from build123d import *

# Parameters (mm, degrees)
F0_W     = 76.2
F0_H     = 76.2
F1_DEPTH = 76.2
F2_T     = -7.62
F3_W     = 60.96
F3_H     = 60.96
F4_DEPTH = 25.4
F5_W     = 60.96
F5_H     = 60.96
F6_DEPTH = 25.4
F7_W     = 60.96
F7_H     = 60.96
F8_DEPTH = 25.4


with BuildPart() as f1:
    # F0 (on Top) → F1 (new body)
    with BuildSketch(Plane.XY):
        with Locations((-3.61854, -0.157197)):
            Rectangle(F0_W, F0_H)
    extrude(amount=F1_DEPTH)

    # F2
    f2_openings = [f1.faces().sort_by_distance(p)[0] for p in [
        (-3.61854, -38.257197, 38.1),
    ]]
    offset(amount=F2_T, openings=f2_openings)

    # F3 (on face) → F4 (cut)
    with BuildSketch(Plane(origin=(-41.71854, 0, 0), x_dir=(0, -1, 0), z_dir=(-1, 0, 0))):
        with Locations((0.157197, 38.1)):
            Rectangle(F3_W, F3_H)
    extrude(amount=-F4_DEPTH, mode=Mode.SUBTRACT)

    # F5 (on face) → F6 (cut)
    with BuildSketch(Plane(origin=(0, 37.942803, 0), x_dir=(-1, 0, 0), z_dir=(0, 1, 0))):
        with Locations((3.61854, 38.1)):
            Rectangle(F5_W, F5_H)
    extrude(amount=-F6_DEPTH, mode=Mode.SUBTRACT)

    # F7 (on face) → F8 (cut)
    with BuildSketch(Plane.YZ.offset(34.48146)):
        with Locations((-0.157197, 38.1)):
            Rectangle(F7_W, F7_H)
    extrude(amount=-F8_DEPTH, mode=Mode.SUBTRACT)


solid = f1.part
CAD build for the part. Positions are in the model's coordinates, mm. A direction names the side the tool comes from. Coordinates: 2 decimals unless noted, no trailing zeros. Order: outer loops, then holes, each group sorted by start corner. A loop starts at its lowest first (then second) coordinate and runs counter-clockwise, first axis right, second up.
Item 1: Band-saw the part on C-C on z = 9.5. List the corners of the cut face in (x, y), plus the area to 3 significant figures.
Check sheet entries:
outline: (-41.72, -38.26) - (-34.1, -38.26) - (-34.1, -30.64) - (-41.72, -30.64) - close; (-41.72, 30.32) - (-34.1, 30.32) - (-34.1, 37.94) - (-41.72, 37.94) - close; (26.86, -38.26) - (34.48, -38.26) - (34.48, -30.64) - (26.86, -30.64) - close; (26.86, 30.32) - (34.48, 30.32) - (34.48, 37.94) - (26.86, 37.94) - close
area: 232 mm2
Item 2: Drill centre lines: L1, parallel to Z at x = -21, y = -16; L2, parallel to X at y = -31.5, z = 30.5; L3, parallel to Y at x = 28, z = 55.5. Where is each one in solid material? Low to high.
Check sheet entries:
L1: z = 0 to 7.62, 68.58 to 76.2
L2: x = -41.72 to -34.1, 26.86 to 34.48
L3: y = -38.26 to -30.64, 30.32 to 37.94
Item 3: Band-saw the part on A-A on y = 11.5. List the corners of the cut face in (x, z).
Check sheet entries:
outline: (-41.72, 0) - (34.48, 0) - (34.48, 7.62) - (-41.72, 7.62) - close; (-41.72, 68.58) - (34.48, 68.58) - (34.48, 76.2) - (-41.72, 76.2) - close
Item 4: 3-axis set-ups, long thin cutter, end or side, ignore diameter. For faces 1 (the face through (-4, 0, 68.58)), 2 (the face through (-38, -30.637, 38)), 3 (the face through (-41.719, -35, 38)), 4 (the face through (-34.099, 34, 38)): which of +Z, -Z, +X, -X, +Y, -Y reach the whole face in a straight line?
Check sheet entries:
face 1: none
face 2: +X, -X
face 3: +Z, -Z, -X, +Y, -Y
face 4: +Y, -Y
Item 5: Band-saw the part on B-B on x = -22.5. List the corners of the cut face in (y, z).
Check sheet entries:
outline: (-38.26, 0) - (37.94, 0) - (37.94, 7.62) - (-38.26, 7.62) - close; (-38.26, 68.58) - (37.94, 68.58) - (37.94, 76.2) - (-38.26, 76.2) - close
Item 6: Two-plate mould, pull along Z, no slides. Class faces 5 (the face through (-38, 30.323, 38)), 6 (the face through (-4, 0, 76.2)), 7 (the face through (-38, 37.943, 38)): +Z half, -Z half, draft (parallel to the pull), parting line (faces both ways), or undercut.
Check sheet entries:
face 5: undercut
face 6: +Z half
face 7: draft
